Read the model definition and answer for the solid it produces. Units are mm, in the model's axes. Give positions to 0.01 mm unless a question says otherwise; leave off trailing zeros. Order: outer loops, then holes, each group sorted by start corner. A loop starts at its lowest first (then second) coordinate and runs counter-clockwise, first axis right, second up. Notation, with made-up numbers: (-7, 56.25) - (15, 56.25) arc R6 ccw to (15, 65.25) - close; hole circle Ø8 at (78.5, 52.25). An arc over 180 degrees is marked (long way). Answer as CSV lines item,"result". Start each with the question number.
from build123d import *

# Parameters (mm, degrees)
BOSS_EXTRU_1_DEPTH = 3
CHANFREIN1_SIZE2   = 5.196152423
CHANFREIN1_SIZE    = 3


with BuildPart() as part:
    # Esquisse1 → Boss.-Extru.1 (new body)
    with BuildSketch(Plane.XY):
        with BuildLine():
            Line((-120, 22.240685392), (-104.948546119, 61.451063305))
            ThreePointArc((-104.948546119, 61.451063305), (0, 42), (104.948546119, 61.451063305))
            Line((104.948546119, 61.451063305), (120, 22.240685392))
            ThreePointArc((120, 22.240685392), (0, 0), (-120, 22.240685392))
        make_face()
    extrude(amount=BOSS_EXTRU_1_DEPTH)

    # Chanfrein1
    chanfrein1_edges = [part.edges().sort_by_distance(p)[0] for p in [
        (0, 0, 3),
    ]]
    chanfrein1_side = [part.faces().sort_by_distance(p)[0] for p in [
        (0, 0, 2.94),
    ]]
    chamfer(chanfrein1_edges, length=CHANFREIN1_SIZE - 0.0001, length2=CHANFREIN1_SIZE2 - 0.0001, reference=chanfrein1_side[0])  # a hair under: the kernel refuses the full size


solid = part.part
(1) Straight lines are drawn through the part: line 1 (Y direction, x = -93, z = 2.25); line 2 (Y direction, x = -77.5, z = 1.5); line 3 (X direction, y = 30, z = 0.35). For each, find the intervals that lie inside material, in ascending order. Write a range as [from, to].
(2) Determine the mould class of faces 1 (the conical face through (1.693, 4.948, 2.854)), 2 (the flat face through (112.37, 42.12, 1.48)), 3 (the flat face through (2, 31, 0)) for opening direction Z: released by +Z, released by -Z, zero draft, split by the parting line, or undercut.
(3) Flat-ended cylindrical pins translate along their axes: pin 1 Ø1.5 at (y, z) = (26, 0.5) entering from +X; pin 2 Ø1.5 at (y, z) = (43, 2) entering from +X; pin 3 Ø8 at (x, y) = (36, 49) entering from -Z. Find the tip coordinate at first contact, or state that the pin passes through.
(4) Section C-C, the plane y = 45.5 is taken. Write down the section's boundary in (x, z), and give its area (3 significant figures).
(5) Section B-B, the plane z = 1.1 is taken. Write down the section's boundary in (x, y), and give its area (3 significant figures).
(6) Section D-D, the plane y = 34 is taken. Write down the section's boundary in (x, z), and give its area (3 significant figures).
Checks:
1,line 1,"y = [17.23, 57.16]"
1,line 2,"y = [11.76, 52.44]"
1,line 3,"x = [-117.02, 117.02]"
2,face 1,"released by +Z"
2,face 2,"zero draft"
2,face 3,"released by -Z"
3,pin 1,"stops at x = 118.84"
3,pin 2,"stops at x = 112.32"
3,pin 3,"passes through"
4,outline,"(-111.07, 0) - (-45.14, 0) - (-45.14, 3) - (-111.07, 3) - close; (45.14, 0) - (111.07, 0) - (111.07, 3) - (45.14, 3) - close"
4,area,"396 mm²"
5,outline,"(-119.32, 24.02) arc R332.95 ccw to (119.32, 24.02) - (104.95, 61.45) arc R292.85 cw to (-104.95, 61.45) - close"
5,area,"9,200 mm²"
6,outline,"(-115.49, 0) - (115.49, 0) - (115.49, 3) - (-115.49, 3) - close"
6,area,"693 mm²"
